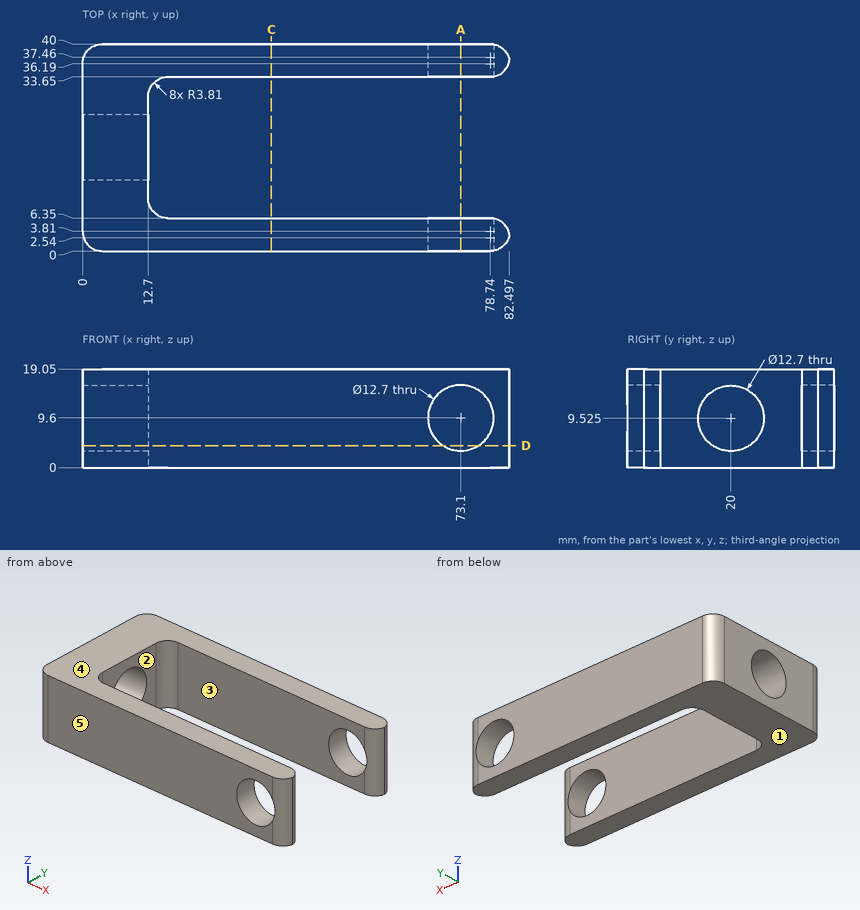
Part print with two shaded views. Sizes in mm from the minimum x, y, z corner. A direction names the side the tool comes from. Give positions to 0.01 mm unless a question says otherwise; leave off trailing zeros. Order: outer loops, then holes, each group sorted by start corner. A loop starts at its lowest first (then second) coordinate and runs counter-clockwise, first axis right, second up.
1) Saw through at A-A, the plane x = 73.1. Write the cut outline in (y, z).
2) Mould opens along Y. For the marked faces 3, 4 and 5 say: +Y half, -Y half, draft (parallel to the pull), parting line (faces both ways), or undercut.
3) Wall check: probe 1 along Y at (x, z) = (28, 5.75); probe 2 along Z at (x, y) = (73.1, 3.5); probe 3 along X at (y, z) = (28.5, 16.25). Give the ranges that are in metal, low to high.
4) Pin check, flat tips, straight feed: pin 1 (1 mm diameter, centred on y = 21.5, z = 4, fed in from -X); pin 2 (2 mm diameter, centred on y = 10.5, z = 12.5, fed in from +X). Stop position of each tip, or through.
5) 3-axis set-ups, long thin cutter, end or side, ignore diameter. For the marked faces 1 and 2: which of +Z, -Z, +X, -X, +Y, -Y reach the whole face in a straight line?
6) Saw through at C-C, the plane x = 36.5. Write the cut outline in (y, z), then the cut area to 3 significant figures.
7) Saw through at D-D, the plane z = 4.25. Count the separate pieces of the cut face and the enclosed holes in it, then the cut area to 3 significant figures.
Computed:
1. outline: (0, 0) - (6.35, 0) - (6.35, 3.25) - (0, 3.25) - close; (0, 15.95) - (6.35, 15.95) - (6.35, 19.05) - (0, 19.05) - close; (33.65, 0) - (40, 0) - (40, 3.25) - (33.65, 3.25) - close; (33.65, 15.95) - (40, 15.95) - (40, 19.05) - (33.65, 19.05) - close
2. face 3: undercut
2. face 4: draft
2. face 5: -Y half
3. probe 1: y = 0 to 6.35, 33.65 to 40
3. probe 2: z = 0 to 3.25, 15.95 to 19.05
3. probe 3: x = 0 to 12.7
4. pin 1: passes through
4. pin 2: stops at x = 12.76
5. face 1: -Z, +X, -X, +Y, -Y
5. face 2: +Z, -Z, +X
6. outline: (0, 0) - (6.35, 0) - (6.35, 19.05) - (0, 19.05) - close; (33.65, 0) - (40, 0) - (40, 19.05) - (33.65, 19.05) - close
6. area: 242 mm2
7. separate pieces: 4
7. enclosed holes: 0
7. area: 1,210 mm2
